Source: CAD feature listing. Evaluate the final solid. Frame: model axes, mm. Give positions to 0.01 mm unless a question says otherwise; leave off trailing zeros. Order: outer loops, then holes, each group sorted by start corner. A loop starts at its lowest first (then second) coordinate and runs counter-clockwise, first axis right, second up.
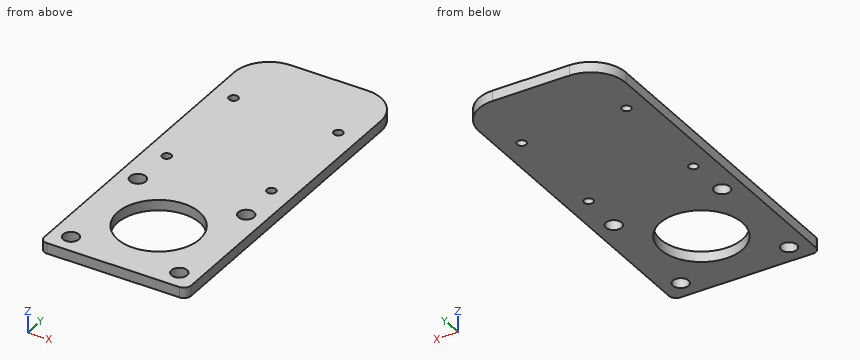
Autodesk Inventor part; units mm, degrees
ref_plane "YZ Plane" through (0, 0, 0) normal (1, 0, 0) x (0, 1, 0)
ref_plane "XZ Plane" through (0, 0, 0) normal (0, 1, 0) x (-1, 0, 0)
ref_plane "XY Plane" through (0, 0, 0) normal (0, 0, 1) x (1, 0, 0)
sketch "スケッチ1" plane through (0, 0, 0) normal (0, 0, 1) x (1, 0, 0)
  line L0 (0, 0) -> (42, 0)
  line L1 (42, 0) -> (42, 100)
  line L2 (42, 100) -> (0, 100)
  line L3 (0, 100) -> (0, 0)
  line L4 (0, 42) -> (42, 42)
  circle A0 centre (5.5, 36.5) radius 2.25
  circle A1 centre (36.5, 36.5) radius 2.25
  circle A2 centre (5.5, 5.5) radius 2.25
  circle A3 centre (36.5, 5.5) radius 2.25
  circle A4 centre (21, 21) radius 11.75
  dimension "d0" = 42
  dimension "d1" = 100
  dimension "d2" = 42
  dimension "d3" = 5.5
  dimension "d4" = 5.5
  dimension "d5" = 5.5
  dimension "d6" = 5.5
  dimension "d7" = 4.5
  dimension "d8" = 4.5
  dimension "d9" = 4.5
  dimension "d10" = 4.5
  dimension "d11" = 23.5
extrude "押し出し1" add sketch "スケッチ1" along normal blind 3
fillet "フィレット1" radius 2 2 edges at (42, 0, 1.5) (0, 0, 1.5)
fillet "フィレット2" radius 10 2 edges at (0, 100, 1.5) (42, 100, 1.5)
sketch "スケッチ2" plane through (0, 0, 3) normal (0, 0, 1) x (1, 0, 0)
  line L0 (0, 90) -> (0, 2)
  line L1 (0, 46) -> (42, 46)
  line L2 (42, 2) -> (42, 90)
  line L3 (0, 52) -> (42, 52)
  line L4 (6, 52) -> (6, 46)
  line L5 (36, 52) -> (36, 46)
  circle A0 centre (6, 49) radius 1.3
  circle A1 centre (36, 49) radius 1.3
  point P0 (0, 0)
  dimension "d16" = 6
  dimension "d17" = 6
  dimension "d18" = 6
  dimension "d19" = 2.6
  dimension "d20" = 2.6
extrude "押し出し2" cut sketch "スケッチ2" against normal blind 3 contours A0 L4 | L4 A0 | A1 L5 | L5 A1
sketch "スケッチ3" plane through (0, 0, 3) normal (0, 0, 1) x (1, 0, 0)
  line L0 (0, 90) -> (0, 2)
  line L1 (0, 46) -> (42, 46)
  line L2 (42, 2) -> (42, 90)
  line L3 (0, 52) -> (42, 52)
  line L4 (6, 52) -> (6, 46)
  line L5 (36, 52) -> (36, 46)
  circle A0 centre (6, 49) radius 1.3
  circle A1 centre (36, 49) radius 1.3
  line L6 (0, 90) -> (0, 2)
  line L7 (0, 77) -> (42, 77)
  line L8 (42, 2) -> (42, 90)
  line L9 (0, 83) -> (42, 83)
  circle A2 centre (6, 80) radius 1.3
  circle A3 centre (36, 80) radius 1.3
  point P0 (0, 0)
  point P1 (0, 0)
  dimension "d23" = 6
  dimension "d24" = 6
  dimension "d25" = 6
  dimension "d26" = 2.6
  dimension "d27" = 2.6
  dimension "d28" = 25
  dimension "d29" = 6
  dimension "d30" = 2.6
  dimension "d31" = 3
  dimension "d32" = 2.6
extrude "押し出し3" cut sketch "スケッチ3" against normal blind 10 contours A2 | A3
1) Section query D-D, the plane y = 27. Return the cut outline in (x, z), and give its area (3 significant figures).
Report:
outline: (0, 0) - (10.9, 0) - (10.9, 3) - (0, 3) - close; (31.1, 0) - (42, 0) - (42, 3) - (31.1, 3) - close
area: 65.4 mm2
2) Section query A-A, the plane x = 21. Return the cut outline in (y, z).
Report:
outline: (0, 0) - (9.25, 0) - (9.25, 3) - (0, 3) - close; (32.75, 0) - (100, 0) - (100, 3) - (32.75, 3) - close
3) Section query C-C, the plane y = 80. Return the cut outline in (x, z).
Report:
outline: (0, 0) - (4.7, 0) - (4.7, 3) - (0, 3) - close; (7.3, 0) - (34.7, 0) - (34.7, 3) - (7.3, 3) - close; (37.3, 0) - (42, 0) - (42, 3) - (37.3, 3) - close
4) Material intervals for L1, parallel to X at y = 49, z = 0.65; L2, parallel to Y at x = 37.5, z = 2; L3, parallel to X at y = 20.5, z = 0.5, sorted ascending.
Report:
L1: x = 0 to 4.7, 7.3 to 34.7, 37.3 to 42
L2: y = 0 to 3.48, 7.52 to 34.48, 38.52 to 98.35
L3: x = 0 to 9.26, 32.74 to 42
5) Section query B-B, the plane z = 0.6. Count the separate pieces of the cut face and the enclosed holes in it, and give its area (3 significant figures).
Report:
separate pieces: 1
enclosed holes: 9
area: 3,640 mm2
